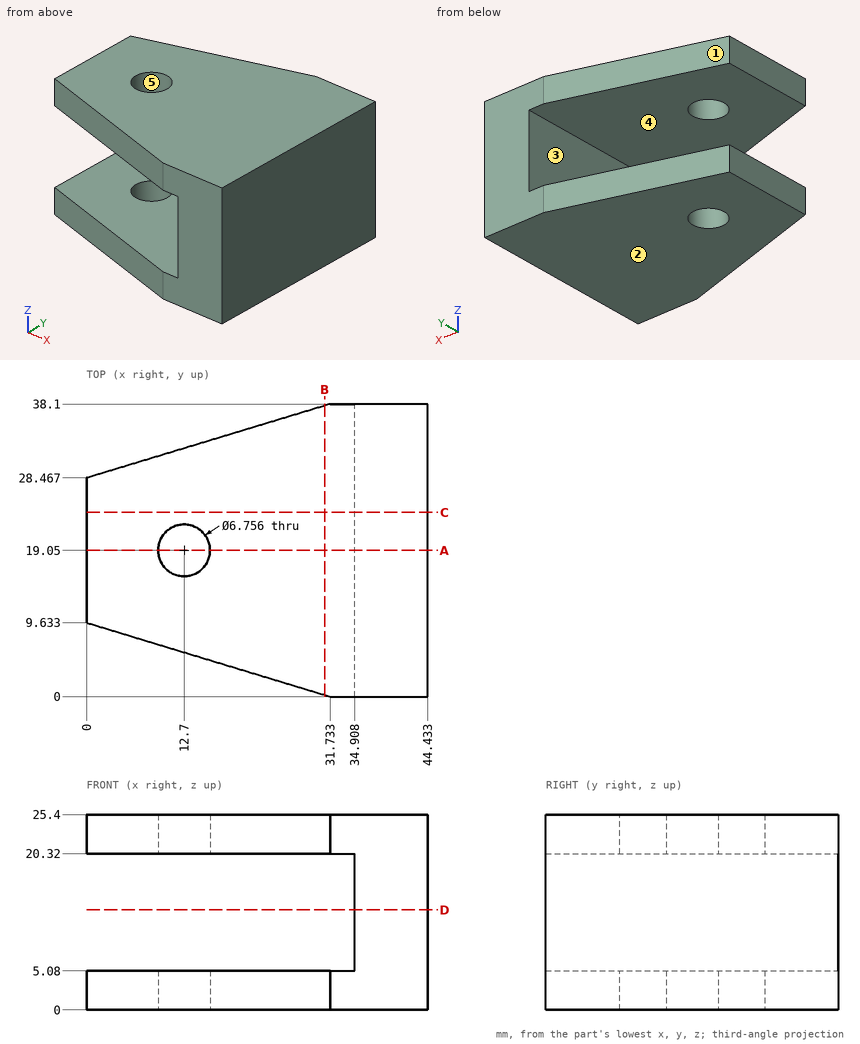
Design review of the part shown in the three views and the two pictorial views. Dimensions are in mm from the part's minimum x, y and z. A direction names the side the tool comes from. Round coordinates to 2 decimals unless told otherwise and drop trailing zeros. Loops run counter-clockwise (first coordinate to the right, second up) from the corner with the lowest first, then second, coordinate; pieces in that order, holes last. Notation, with made-up numbers: (-27.75, 20) -> (-1.75, 20) arc R27 ccw to (-1.75, 44) -> close; hole circle Ø5 at (-23.5, 36.25). An arc over 180 degrees is marked (long way). Use one line per item in the form item = value. Start each with the question number.
Q1. Draft analysis for pull direction Z (two halves, no side actions). For the marked faces 1, 2 and 3, state which applies: +Z half, -Z half, draft (parallel to the pull), parting line (faces both ways), or undercut.
Q2. Wall thickness on line 1 along Z through (x, y) = (27.5, 24.5); line 2 along X through (y, z) = (19.05, 3.75); line 3 along X through (y, z) = (22, 7.75): over which ranges is each line inside the solid? List them lowest first. Write a range as [from, to].
Q3. We need section C-C on y = 24. Give the boundary of the cut face in (x, z).
Q4. For pin 1 Ø1 at (x, z) = (34, 13.5) entering from -Y; pin 2 Ø6 at (x, z) = (17, 5.5) entering from +Y, all flat-tipped, find the tip position at first contact; note any pin that passes through.
Q5. We need section B-B on x = 31. Give the boundary of the cut face in (y, z).
Q6. Machinability: for the marked faces 4 and 5, which of the approach directions +Z, -Z, +X, -X, +Y, -Y give a long, thin tool a straight path to every point of the face, cutting with its end or side? Answer none if there is none.
Q7. We need section A-A on y = 19.05. Give the boundary of the cut face in (x, z), then the cut area to 3 significant figures.
Q8. We need section D-D on z = 13. Give the boundary of the cut face in (x, y), then the cut area to 3 significant figures.
Calculated:
q1.face_1 = draft
q1.face_2 = -Z half
q1.face_3 = undercut
q2.line_1 = [0, 5.08], [20.32, 25.4]
q2.line_2 = [0, 9.32], [16.08, 44.43]
q2.line_3 = [34.91, 44.43]
q3.outline = (0, 0) -> (44.43, 0) -> (44.43, 25.4) -> (0, 25.4) -> (0, 20.32) -> (34.91, 20.32) -> (34.91, 5.08) -> (0, 5.08) -> close
q4.pin_1 = through
q4.pin_2 = 34.53
q5.outline = (0.22, 0) -> (37.88, 0) -> (37.88, 5.08) -> (0.22, 5.08) -> close; (0.22, 20.32) -> (37.88, 20.32) -> (37.88, 25.4) -> (0.22, 25.4) -> close
q6.face_4 = -X, +Y, -Y
q6.face_5 = +Z, -Z
q7.outline = (0, 0) -> (9.32, 0) -> (9.32, 5.08) -> (0, 5.08) -> close; (0, 20.32) -> (9.32, 20.32) -> (9.32, 25.4) -> (0, 25.4) -> close; (16.08, 0) -> (44.43, 0) -> (44.43, 25.4) -> (16.08, 25.4) -> (16.08, 20.32) -> (34.91, 20.32) -> (34.91, 5.08) -> (16.08, 5.08) -> close
q7.area = 528 mm²
q8.outline = (34.91, 0) -> (44.43, 0) -> (44.43, 38.1) -> (34.91, 38.1) -> close
q8.area = 363 mm²
